```python
from build123d import *

# Parameters (mm, degrees)
SKETCH3_R           = 6.5
SKETCH3_R_2         = 11.5
BOSS_EXTRUDE2_DEPTH = 3.5
BOSS_EXTRUDE3_START = 1.5
SKETCH4_R           = 8
SKETCH4_R_2         = 4.5
BOSS_EXTRUDE3_DEPTH = 1.5
SKETCH6_R           = 7
BOSS_EXTRUDE4_DEPTH = 16
CUT_EXTRUDE1_START  = -3.5
CUT_EXTRUDE1_DEPTH  = 3.5
SKETCH8_R           = 1.575
CUT_EXTRUDE2_DEPTH  = 3


with BuildPart() as part:
    # Sketch3 → Boss-Extrude2 (new body)
    with BuildSketch(Plane(origin=(0, 20, 0), x_dir=(0, 1, 0), z_dir=(-1, 0, 0))):
        with BuildLine():
            Line((-3.5, 101.628977271), (-3.5, -57.9976886))
            ThreePointArc((-3.5, -57.9976886), (-20, -74.4976886), (-36.5, -57.9976886))
            Line((-36.5, -57.9976886), (-36.5, 101.628977271))
            ThreePointArc((-36.5, 101.628977271), (-20, 118.128977271), (-3.5, 101.628977271))
        make_face()
        with Locations(Location((-20, 0, 0), (0, 0, 270))):
            Circle(SKETCH3_R, mode=Mode.SUBTRACT)
        with Locations(Location((-20, -57.9976886, 0), (0, 0, 270))):
            Circle(SKETCH3_R_2, mode=Mode.SUBTRACT)
    extrude(amount=BOSS_EXTRUDE2_DEPTH)

    # Sketch4 → Boss-Extrude3 (add)
    with BuildSketch(Plane(origin=(0, 0, 0), x_dir=(0, 0, -1), z_dir=(1, 0, 0)).offset(BOSS_EXTRUDE3_START)):
        with BuildLine():
            Line((101.628977271, 16.5), (-57.9976886, 16.5))
            ThreePointArc((-57.9976886, 16.5), (-74.4976886, 0), (-57.9976886, -16.5))
            Line((-57.9976886, -16.5), (101.628977271, -16.5))
            ThreePointArc((101.628977271, -16.5), (118.128977271, 0), (101.628977271, 16.5))
        make_face()
        with Locations((-57.9976886, 0)):
            Circle(SKETCH4_R, mode=Mode.SUBTRACT)
        Circle(SKETCH4_R_2, mode=Mode.SUBTRACT)
    extrude(amount=-BOSS_EXTRUDE3_DEPTH)

    # Sketch6 → Boss-Extrude4 (add)
    with BuildSketch(Plane(origin=(1.5, 0, 0), x_dir=(0, 0, -1), z_dir=(1, 0, 0))):
        with Locations((101.628977271, 0)):
            Circle(SKETCH6_R)
    extrude(amount=BOSS_EXTRUDE4_DEPTH)

    # Sketch7 → Cut-Extrude1 (cut)
    with BuildSketch(Plane.ZY.offset(3.5).offset(CUT_EXTRUDE1_START)):
        with BuildLine():
            Line((-2, 16.5), (-2, 6.184658438))
            ThreePointArc((-2, 6.184658438), (0, 6.5), (2, 6.184658438))
            Line((2, 6.184658438), (2, 16.5))
            Line((2, 16.5), (-2, 16.5))
        make_face()
    extrude(amount=CUT_EXTRUDE1_DEPTH, mode=Mode.SUBTRACT)

    # Sketch8 → Cut-Extrude2 (cut)
    with BuildSketch(Plane.XY.offset(-94.628977271)):
        with Locations((14.925, 0)):
            Circle(SKETCH8_R)
    cut_extrude2 = extrude(amount=-CUT_EXTRUDE2_DEPTH, mode=Mode.SUBTRACT)

    # Mirror1: Cut-Extrude2 across plane
    add(cut_extrude2.mirror(Plane.XY.offset(-101.628977271)), mode=Mode.SUBTRACT)


solid = part.part
```
Design review of the part built by this model. Coordinates are the model's own, in mm. A direction names the side the tool comes from. Give positions to 0.01 mm unless a question says otherwise; leave off trailing zeros. Write each loop counter-clockwise with the first axis right and the second up, starting at its lowest first coordinate (ties: lowest second). Pieces come first, ordered by that corner, then holes. Notation, with made-up numbers: (0.25, 37) -> (14.25, 37) arc R25 cw to (14.25, 56) -> close; hole circle Ø11 at (89, 46.25). An arc over 180 degrees is marked (long way). Answer in a Markdown table with one row per item.
(1) Consider section D-D (z = 32). State the section outline as (x, y) points, then the cut area to 3 significant figures.
Results:
| item | result |
|---|---|
| outline | (-3.5, -16.5) -> (1.5, -16.5) -> (1.5, 16.5) -> (-3.5, 16.5) -> close |
| area | 165 mm2 |
(2) Consider section C-C (x = 9). State the section outline as (y, z) points, then the cut area to 3 significant figures.
Results:
| item | result |
|---|---|
| outline | circle Ø14 at (0, -101.63) |
| area | 154 mm2 |
(3) Consider section B-B (y = 0). Count the separate pieces of the cut face and the enclosed holes in it, then the cut area to 3 significant figures.
Results:
| item | result |
|---|---|
| separate pieces | 3 |
| enclosed holes | 0 |
| area | 1,000 mm2 |
(4) For faces 1 (the flat face through (15, 0, -97.629)), 2 (the cylindrical face through (16.43, 0.47, -107.15)), 3 (the cylindrical face through (9.388, 2.103, -108.306)), 4 (the flat face through (-2, 11, 2)), list the 3-axis set-ups (+Z, -Z, +X, -X, +Y, -Y) from which the entire face can be reached by the end or side of a thin tool; tool diameter is ignored.
Results:
| item | result |
|---|---|
| face 1 | +Z |
| face 2 | -Z |
| face 3 | +X |
| face 4 | -X, +Y |
(5) Mouldability with a two-part tool opening along Z and no side actions: class faces 5 (the cylindrical face through (-0.965, 0.363, 74.494)), 6 (the cylindrical face through (16.43, 0.47, -96.11)), 7 (the flat face through (0, 5, 0)) as +Z half, -Z half, draft (parallel to the pull), parting line (faces both ways), or undercut.
Results:
| item | result |
|---|---|
| face 5 | +Z half |
| face 6 | draft |
| face 7 | undercut |
(6) To check wall thickness, follow probe 1 along Y at (x, z) = (0.4, 0); probe 2 along X at (y, z) = (0, -96); probe 3 along X at (y, z) = (-5.5, -11.5). State the ranges of each line that lie inside material, in increasing order.
Results:
| item | result |
|---|---|
| probe 1 | -16.5 to -4.5, 4.5 to 16.5 |
| probe 2 | -3.5 to 13.35, 16.5 to 17.5 |
| probe 3 | -3.5 to 1.5 |
(7) Consider section A-A (z = 0). State the section outline as (x, y) points.
Results:
| item | result |
|---|---|
| outline | (-3.5, -16.5) -> (1.5, -16.5) -> (1.5, -4.5) -> (0, -4.5) -> (0, -6.5) -> (-3.5, -6.5) -> close; (0, 4.5) -> (1.5, 4.5) -> (1.5, 16.5) -> (0, 16.5) -> close |
(8) Clearance check with flat-ended pins moving along their axes: pin 1 (3 mm diameter, centred on x = 14.925, y = 0, fed in from +Z); pin 2 (1 mm diameter, centred on x = -1.5, y = 9, fed in from -Z); pin 3 (18.5 mm diameter, centred on y = 0, z = 58, fed in from -X); pin 4 (1 mm diameter, centred on x = 3.5, y = -11, fed in from -Z). State where each tip first meets the part, or that it passes through.
Results:
| item | result |
|---|---|
| pin 1 | z = -97.63 |
| pin 2 | z = -115.77 |
| pin 3 | x = 0 |
| pin 4 | through |
